```python
from build123d import *

# Parameters (mm, degrees)
SKETCH1_W           = 115
SKETCH1_H           = 50
BOSS_EXTRUDE1_DEPTH = 8
SKETCH2_R           = 4
CUT_EXTRUDE1_DEPTH  = 10
CUT_EXTRUDE2_DEPTH  = 5
LPATTERN1_COUNT     = 2
LPATTERN1_PITCH     = 37
CUT_EXTRUDE3_DEPTH  = 3
CUT_EXTRUDE4_DEPTH  = 23
CUT_EXTRUDE8_DEPTH  = 5
CUT_EXTRUDE9_DEPTH  = 5


with BuildPart() as part:
    # Sketch1 → Boss-Extrude1 (new body)
    with BuildSketch(Plane(origin=(0, 0, 0), x_dir=(1, 0, 0), z_dir=(0, 1, 0))):
        Rectangle(SKETCH1_W, SKETCH1_H)
    extrude(amount=BOSS_EXTRUDE1_DEPTH)

    # Sketch2 → Cut-Extrude1 (cut)
    with BuildSketch(Plane(origin=(0, 8, 0), x_dir=(1, 0, 0), z_dir=(0, 1, 0))):
        with Locations(Location((-40.5, 0, 0), (0, 0, 270))):
            Circle(SKETCH2_R)
    extrude(amount=-CUT_EXTRUDE1_DEPTH, mode=Mode.SUBTRACT)

    # Sketch3 → Cut-Extrude2 (cut)
    with BuildSketch(Plane(origin=(0, 8, 0), x_dir=(1, 0, 0), z_dir=(0, 1, 0))):
        with BuildLine():
            Line((-29, -10.5), (-29, 10.5))
            ThreePointArc((-29, 10.5), (-26, 13.5), (-23, 10.5))
            Line((-23, 10.5), (-23, -10.5))
            ThreePointArc((-23, -10.5), (-26, -13.5), (-29, -10.5))
        make_face()
    cut_extrude2 = extrude(amount=-CUT_EXTRUDE2_DEPTH, mode=Mode.SUBTRACT)

    # LPattern1: Cut-Extrude2 ×2
    with Locations(*[(i * LPATTERN1_PITCH, 0, 0) for i in range(1, LPATTERN1_COUNT)]):
        add(cut_extrude2, mode=Mode.SUBTRACT)

    # Sketch4 → Cut-Extrude3 (cut)
    with BuildSketch(Plane(origin=(0, 8, 0), x_dir=(1, 0, 0), z_dir=(0, 1, 0))):
        with BuildLine():
            Line((34, 15), (34, -15))
            ThreePointArc((34, -15), (32, -17), (30, -15))
            Line((30, -15), (30, 15))
            ThreePointArc((30, 15), (32, 17), (34, 15))
        make_face()
    extrude(amount=-CUT_EXTRUDE3_DEPTH, mode=Mode.SUBTRACT)

    # Sketch5 → Cut-Extrude4 (cut)
    with BuildSketch(Plane(origin=(57.5, 0, 0), x_dir=(0, 0, -1), z_dir=(1, 0, 0))):
        with BuildLine():
            Line((11.66190379, 8), (0, 23))
            Line((0, 23), (-11.66190379, 8))
            ThreePointArc((-11.66190379, 8), (0, 4), (11.66190379, 8))
        make_face()
    extrude(amount=-CUT_EXTRUDE4_DEPTH, mode=Mode.SUBTRACT)

    # Sketch9 → Cut-Extrude8 (cut)
    with BuildSketch(Plane.XZ):
        with BuildLine():
            Line((-8.787415011, 3.25), (-6.212584989, 3.25))
            ThreePointArc((-6.212584989, 3.25), (-4.573205347, 2.926794653), (-4.25, 1.287415011))
            Line((-4.25, 1.287415011), (-4.25, -1.287415011))
            ThreePointArc((-4.25, -1.287415011), (-4.573205347, -2.926794653), (-6.212584989, -3.25))
            Line((-6.212584989, -3.25), (-8.787415011, -3.25))
            ThreePointArc((-8.787415011, -3.25), (-10.426794653, -2.926794653), (-10.75, -1.287415011))
            Line((-10.75, -1.287415011), (-10.75, 1.287415011))
            ThreePointArc((-10.75, 1.287415011), (-10.426794653, 2.926794653), (-8.787415011, 3.25))
        make_face()
    extrude(amount=-CUT_EXTRUDE8_DEPTH, mode=Mode.SUBTRACT)

    # Sketch10 → Cut-Extrude9 (cut)
    with BuildSketch(Plane.XZ):
        with BuildLine():
            ThreePointArc((2.399494937, 9.899494937), (-20.434313455, 5.357568053), (-7.5, -14))
            ThreePointArc((-7.5, -14), (-5.5, -12), (-7.5, -10))
            ThreePointArc((-7.5, -10), (-16.738795325, 3.826834324), (-0.428932188, 7.071067812))
            ThreePointArc((-0.428932188, 7.071067812), (2.399494937, 7.071067812), (2.399494937, 9.899494937))
        make_face()
    extrude(amount=-CUT_EXTRUDE9_DEPTH, mode=Mode.SUBTRACT)


solid = part.part
```
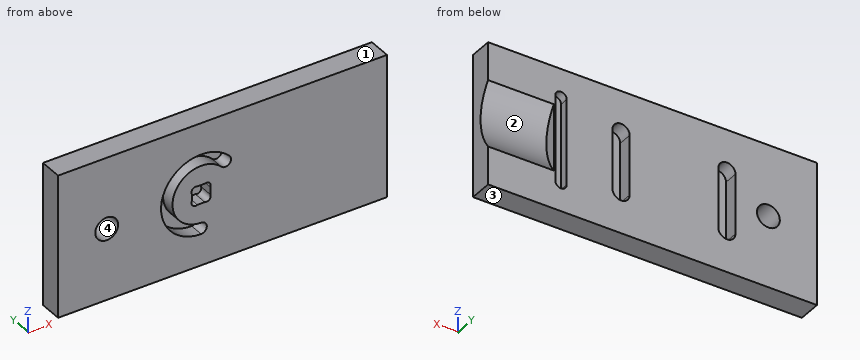
Geometry: final body of the model. Coordinates: model frame, mm. Face numbers are marked on the shaded views. Coordinates: 2 decimals unless noted, no trailing zeros. Order: outer loops, then holes, each group sorted by start corner. A loop starts at its lowest first (then second) coordinate and runs counter-clockwise, first axis right, second up. Notation, with made-up numbers: (69.25, 8.25) -> (113.25, 8.25) arc R23 ccw to (113.25, 44.25) -> close; hole circle Ø4 at (78.5, 54). An arc over 180 degrees is marked (long way). Answer in a Markdown table with one row per item.
Item 1: Section D-D on y = 1.5. Output: boundary loops of the cut face in (x, z).
Return value:
| item | result |
|---|---|
| outline | (-57.5, -25) -> (57.5, -25) -> (57.5, 25) -> (-57.5, 25) -> close; hole circle Ø8 at (-40.5, 0); hole (-10.75, -1.29) arc R1.5 ccw to (-8.79, -3.25) -> (-6.21, -3.25) arc R1.5 ccw to (-4.25, -1.29) -> (-4.25, 1.29) arc R1.5 ccw to (-6.21, 3.25) -> (-8.79, 3.25) arc R1.5 ccw to (-10.75, 1.29) -> close; hole (-7.5, -14) arc R2 ccw to (-7.5, -10) arc R10 cw (long way) to (-0.43, 7.07) arc R2 ccw to (2.4, 9.9) arc R14 ccw (long way) to start |
Item 2: Section A-A on x = -40.5. Output: boundary loops of the cut face in (y, z), plus the area to 3 significant figures.
Return value:
| item | result |
|---|---|
| outline | (0, -25) -> (8, -25) -> (8, -4) -> (0, -4) -> close; (0, 4) -> (8, 4) -> (8, 25) -> (0, 25) -> close |
| area | 336 mm² |
Item 3: Section C-C on x = 32. Output: boundary loops of the cut face in (y, z), plus the area to 3 significant figures.
Return value:
| item | result |
|---|---|
| outline | (0, -25) -> (8, -25) -> (8, -17) -> (5, -17) -> (5, 17) -> (8, 17) -> (8, 25) -> (0, 25) -> close |
| area | 298 mm² |
Item 4: Contact query for flat-ended pins moving along their axis: P1, Ø2, axis at x = -7, z = 0, coming from the -Y side; P2, Ø2.5, axis at y = 6.5, z = 4.5, coming from the +X side; P3, Ø2, axis at x = 32.5, z = -1.5, coming from the +Y side. Output: stop coordinate, or through.
Return value:
| item | result |
|---|---|
| P1 | stops at y = 5 |
| P2 | stops at x = 34.5 |
| P3 | stops at y = 5 |
Item 5: Draft query along Z for the marked faces 1, 2, 3 and 4. Return one class per face: released by +Z, released by -Z, zero draft, split by the parting line, or undercut.
Return value:
| item | result |
|---|---|
| face 1 | released by +Z |
| face 2 | undercut |
| face 3 | released by -Z |
| face 4 | undercut |
Item 6: Ray query, L1, parallel to Z at x = -7.5, y = 1; L2, parallel to X at y = 5.5, z = 0; L3, parallel to X at y = 5.5, z = -4.5. Return the intervals inside material, ascending.
Return value:
| item | result |
|---|---|
| L1 | z = -25 to -14, -10 to -3.25, 3.25 to 10, 14 to 25 |
| L2 | x = -57.5 to -44.5, -36.5 to -29, -23 to 8, 14 to 30, 34 to 34.5 |
| L3 | x = -57.5 to -29, -23 to 8, 14 to 30, 34 to 34.5 |
